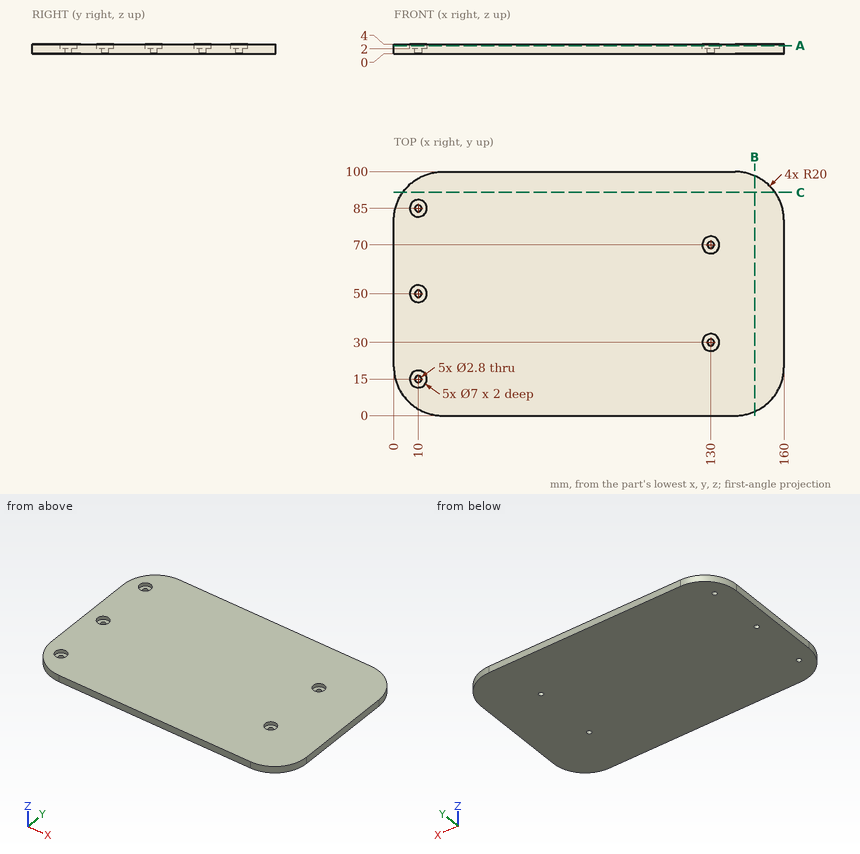
Design review of the part shown in the three views and the two pictorial views. Dimensions are in mm from the part's minimum x, y and z. Round coordinates to 2 decimals unless told otherwise and drop trailing zeros. Loops run counter-clockwise (first coordinate to the right, second up) from the corner with the lowest first, then second, coordinate; pieces in that order, holes last.
(1) Clearance check with flat-ended pins moving along their axes: P1, Ø2, axis at x = 9, y = 85, coming from the +Z side; P2, Ø2, axis at x = 10, y = 15, coming from the -Z side. State where each tip first meets the part, or that it passes through.
Returned:
P1: stops at z = 2
P2: passes through
(2) Wall thickness on line 1 along Y through (x, z) = (10, 1.4); line 2 along X through (y, z) = (87, 2.7) (3 decimals); line 3 along X through (y, z) = (18, 1.3): over which ranges is each line inside the solid? List them lowest first.
Returned:
line 1: y = 2.68 to 13.6, 16.4 to 48.6, 51.4 to 83.6, 86.4 to 97.32
line 2: x = 1.265 to 7.128, 12.872 to 158.735
line 3: x = 0.1 to 159.9
(3) We need section B-B (x = 148). Give the boundary of the cut face in (y, z).
Returned:
outline: (1.67, 0) - (98.33, 0) - (98.33, 4) - (1.67, 4) - close
(4) We need section C-C (y = 91.5). Give the boundary of the cut face in (x, z), plus the area to 3 significant figures.
Returned:
outline: (3.64, 0) - (156.36, 0) - (156.36, 4) - (3.64, 4) - close
area: 611 mm2
(5) We need section A-A (z = 3.3). Give the boundary of the cut face in (x, y), plus the area to 3 significant figures.
Returned:
outline: (0, 20) arc R20 ccw to (20, 0) - (140, 0) arc R20 ccw to (160, 20) - (160, 80) arc R20 ccw to (140, 100) - (20, 100) arc R20 ccw to (0, 80) - close; hole circle Ø7 at (10, 15); hole circle Ø7 at (10, 50); hole circle Ø7 at (10, 85); hole circle Ø7 at (130, 30); hole circle Ø7 at (130, 70)
area: 15,500 mm2
